```python
from build123d import *

# Parameters (mm, degrees)
SKETCH1_W           = 67
SKETCH1_H           = 60
SKETCH1_R           = 2
BOSS_EXTRUDE1_DEPTH = 3
SKETCH2_W           = 67
SKETCH2_H           = 3
BOSS_EXTRUDE2_DEPTH = 57
FILLET1_R           = 33.5
SKETCH3_R           = 10
SKETCH3_R_2         = 1.5
CUT_EXTRUDE1_DEPTH  = 57
BOSS_EXTRUDE3_DEPTH = 1
BOSS_EXTRUDE4_START = -66
BOSS_EXTRUDE4_DEPTH = 1


with BuildPart() as part:
    # Sketch1 → Boss-Extrude1 (new body)
    with BuildSketch(Plane.XY):
        Rectangle(SKETCH1_W, SKETCH1_H)
        with Locations((-28.5, 18.516649199)):
            Circle(SKETCH1_R, mode=Mode.SUBTRACT)
        with Locations(Location((28.5, 18.516649199, 0), (0, 0, 180))):
            Circle(SKETCH1_R, mode=Mode.SUBTRACT)
        with Locations((28.5, -18.516649199)):
            Circle(SKETCH1_R, mode=Mode.SUBTRACT)
        with Locations(Location((-28.5, -18.516649199, 0), (0, 0, 180))):
            Circle(SKETCH1_R, mode=Mode.SUBTRACT)
    extrude(amount=BOSS_EXTRUDE1_DEPTH)

    # Sketch2 → Boss-Extrude2 (add)
    with BuildSketch(Plane.XY.offset(3)):
        with Locations((0, -28.5)):
            Rectangle(SKETCH2_W, SKETCH2_H)
    extrude(amount=BOSS_EXTRUDE2_DEPTH)

    # Fillet1
    fillet1_edges = [part.edges().sort_by_distance(p)[0] for p in [
        (-33.5, -28.5, 60),
        (33.5, -28.5, 60),
    ]]
    fillet(fillet1_edges, radius=FILLET1_R - 0.0001)  # a hair under: the kernel refuses the full size

    # Sketch3 → Cut-Extrude1 (cut)
    with BuildSketch(Plane.XZ.offset(30)):
        with Locations(Location((0, 26.5, 0), (0, 0, 270))):
            Circle(SKETCH3_R)
        with Locations(Location((0, 42.252397405, 0), (0, 0, 270))):
            Circle(SKETCH3_R_2)
        with Locations(Location((11.138627025, 37.638627025, 0), (0, 0, 270))):
            Circle(SKETCH3_R_2)
        with Locations(Location((15.752397405, 26.5, 0), (0, 0, 270))):
            Circle(SKETCH3_R_2)
        with Locations(Location((11.138627025, 15.361372975, 0), (0, 0, 270))):
            Circle(SKETCH3_R_2)
        with Locations(Location((0, 10.747602595, 0), (0, 0, 270))):
            Circle(SKETCH3_R_2)
        with Locations(Location((-11.138627025, 15.361372975, 0), (0, 0, 270))):
            Circle(SKETCH3_R_2)
        with Locations(Location((-15.752397405, 26.5, 0), (0, 0, 270))):
            Circle(SKETCH3_R_2)
        with Locations(Location((-11.138627025, 37.638627025, 0), (0, 0, 270))):
            Circle(SKETCH3_R_2)
    extrude(amount=-CUT_EXTRUDE1_DEPTH, mode=Mode.SUBTRACT)

    # Sketch4 → Boss-Extrude3 (add)
    with BuildSketch(Plane.ZY.offset(33.5)):
        Polygon((3, -2), (18, -27), (3, -27), align=None)
    extrude(amount=-BOSS_EXTRUDE3_DEPTH)

    # Sketch4<2> → Boss-Extrude4 (add)
    with BuildSketch(Plane.ZY.offset(33.5).offset(BOSS_EXTRUDE4_START)):
        Polygon((3, -2), (18, -27), (3, -27), align=None)
    extrude(amount=-BOSS_EXTRUDE4_DEPTH)


solid = part.part
```
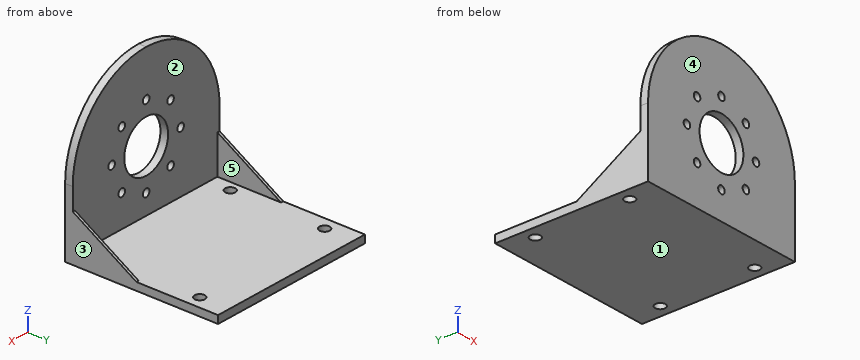
The listing builds one solid part. Answer for the finished solid, in the listing's coordinates (mm). Face numbers are marked on the shaded views. A direction names the side the tool comes from. Round coordinates to 2 decimals unless told otherwise and drop trailing zeros. Write each loop counter-clockwise with the first axis right and the second up, starting at its lowest first coordinate (ties: lowest second). Pieces come first, ordered by that corner, then holes. Notation, with made-up numbers: (27.25, 61) -> (70.25, 61) arc R14 cw to (70.25, 70) -> close; hole circle Ø6 at (21, 18.5). An arc over 180 degrees is marked (long way). Write item = value, one per line.
1) Straight lines are drawn through the part: line 1 along X through (y, z) = (-28.05, 26.5); line 2 along Y through (x, z) = (-2, 45); line 3 along Z through (x, y) = (21.5, -24). For each, find the intervals that lie inside material, in ascending order. Write a range as [from, to].
Check values:
line_1 = [-33.5, -17.25], [-14.25, -10], [10, 14.25], [17.25, 33.5]
line_2 = [-30, -27]
line_3 = [0, 3]
2) Section A-A on x = -28.5 is taken. Write down the section's boundary in (y, z).
Check values:
outline = (-30, 0) -> (-20.52, 0) -> (-20.52, 3) -> (-27, 3) -> (-27, 44.11) -> (-30, 44.11) -> close; (-16.52, 0) -> (16.52, 0) -> (16.52, 3) -> (-16.52, 3) -> close; (20.52, 0) -> (30, 0) -> (30, 3) -> (20.52, 3) -> close
3) Section B-B on z = 31.5 is taken. Write down the section's boundary in (x, y), plus the area to 3 significant figures.
Check values:
outline = (-33.12, -30) -> (-8.66, -30) -> (-8.66, -27) -> (-33.12, -27) -> close; (8.66, -30) -> (33.12, -30) -> (33.12, -27) -> (8.66, -27) -> close
area = 147 mm²
4) Which of the six approach directions +Z, -Z, +X, -X, +Y, -Y give full straight-line access (tool end or side, diameter ignored) to the marked faces 1 and 2?
Check values:
face_1 = -Z, +X, -X, +Y, -Y
face_2 = +Z, +Y
5) Given pin 1 (1 mm diameter, centred on x = 26.5, z = 25, fed in from +Y); pin 2 (4 mm diameter, centred on x = -25.5, y = -22, fed in from +Z), each flat-ended and moving along its own axis, determine where each tip first touches the part or whether it passes through.
Check values:
pin_1 = -27
pin_2 = 3
6) Section D-D on y = 23 is taken. Write down the section's boundary in (x, z), plus the area to 3 significant figures.
Check values:
outline = (-33.5, 0) -> (33.5, 0) -> (33.5, 3) -> (-33.5, 3) -> close
area = 201 mm²
7) Section C-C on x = 8 is taken. Write down the section's boundary in (y, z), plus the area to 3 significant figures.
Check values:
outline = (-30, 0) -> (30, 0) -> (30, 3) -> (-27, 3) -> (-27, 20.5) -> (-30, 20.5) -> close; (-30, 32.5) -> (-27, 32.5) -> (-27, 59.03) -> (-30, 59.03) -> close
area = 312 mm²
8) For a pull along X with two mould halves and no side action, classify the marked faces 3, 4 and 5 as released by +X, released by -X, zero draft, split by the parting line, or undercut.
Check values:
face_3 = released by +X
face_4 = zero draft
face_5 = undercut
